```python
from build123d import *

# Parameters (mm, degrees)
SKETCH1_R               = 11.5
SKETCH1_R_2             = 10
BOSS_EXTRUDE1_DEPTH     = 6
SKETCH2_R               = 6
BOSS_EXTRUDE3_DEPTH     = 18
SKETCH4_R               = 10
CUT_EXTRUDE2_DEPTH      = 7.000000123
CUT_EXTRUDE2_DEPTH_BACK = 7.000000101
SKETCH5_R               = 4
CUT_EXTRUDE3_DEPTH      = 10
SKETCH6_R               = 4.5
SKETCH6_R_2             = 3
BOSS_EXTRUDE4_DEPTH     = 5
SKETCH7_R               = 4
CUT_EXTRUDE4_DEPTH      = 10
BOSS_EXTRUDE5_DEPTH     = 21
SKETCH9_R               = 10
CUT_EXTRUDE5_DEPTH      = 1.0000001
CUT_EXTRUDE5_DEPTH_BACK = 15.0000001
SKETCH10_R              = 1.5
CUT_EXTRUDE6_DEPTH      = 8


with BuildPart() as part:
    # Sketch1 → Boss-Extrude1 (new body, symmetric)
    with BuildSketch(Plane.XY):
        Circle(SKETCH1_R)
        Circle(SKETCH1_R_2, mode=Mode.SUBTRACT)
    extrude(amount=BOSS_EXTRUDE1_DEPTH, both=True)

    # Sketch2 → Boss-Extrude3 (add)
    with BuildSketch(Plane(origin=(0, 25, 0), x_dir=(1, 0, 0), z_dir=(0, 1, 0))):
        Circle(SKETCH2_R)
    extrude(amount=-BOSS_EXTRUDE3_DEPTH)

    # Sketch4 → Cut-Extrude2 (cut, two sides)
    with BuildSketch(Plane.XY) as cut_extrude2_sk:
        Circle(SKETCH4_R)
    extrude(amount=CUT_EXTRUDE2_DEPTH, mode=Mode.SUBTRACT)
    extrude(cut_extrude2_sk.sketch, amount=-CUT_EXTRUDE2_DEPTH_BACK, mode=Mode.SUBTRACT)

    # Sketch5 → Cut-Extrude3 (cut)
    with BuildSketch(Plane(origin=(0, 25, 0), x_dir=(1, 0, 0), z_dir=(0, 1, 0))):
        Circle(SKETCH5_R)
    extrude(amount=-CUT_EXTRUDE3_DEPTH, mode=Mode.SUBTRACT)

    # Sketch6 → Boss-Extrude4 (add)
    with BuildSketch(Plane.XY.offset(8)):
        with Locations((0, 19)):
            Circle(SKETCH6_R)
        with Locations((0, 19)):
            Circle(SKETCH6_R_2, mode=Mode.SUBTRACT)
    extrude(amount=-BOSS_EXTRUDE4_DEPTH)

    # Sketch7 → Cut-Extrude4 (cut)
    with BuildSketch(Plane(origin=(0, 25, 0), x_dir=(1, 0, 0), z_dir=(0, 1, 0))):
        Circle(SKETCH7_R)
    extrude(amount=-CUT_EXTRUDE4_DEPTH, mode=Mode.SUBTRACT)

    # Sketch8 → Boss-Extrude5 (add)
    with BuildSketch(Plane(origin=(0, 25, 0), x_dir=(1, 0, 0), z_dir=(0, 1, 0))):
        with BuildLine():
            Line((-1.5, -3.708099244), (1.5, -3.708099244))
            ThreePointArc((1.5, -3.708099244), (0, -4), (-1.5, -3.708099244))
        make_face()
    extrude(amount=-BOSS_EXTRUDE5_DEPTH)

    # Sketch9 → Cut-Extrude5 (cut, two sides)
    with BuildSketch(Plane.XY.offset(8)) as cut_extrude5_sk:
        Circle(SKETCH9_R)
    extrude(amount=CUT_EXTRUDE5_DEPTH, mode=Mode.SUBTRACT)
    extrude(cut_extrude5_sk.sketch, amount=-CUT_EXTRUDE5_DEPTH_BACK, mode=Mode.SUBTRACT)

    # Sketch10 → Cut-Extrude6 (cut)
    with BuildSketch(Plane.XY.offset(8)):
        with Locations((0, 19)):
            Circle(SKETCH10_R)
    extrude(amount=-CUT_EXTRUDE6_DEPTH, mode=Mode.SUBTRACT)


solid = part.part
```
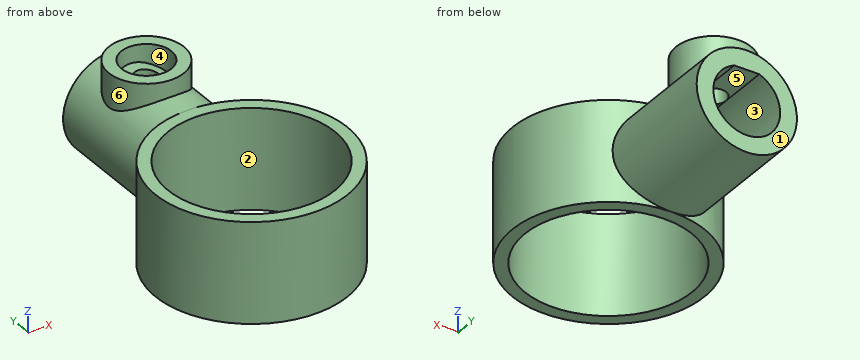
Design review of the part built by this model. Coordinates are the model's own, in mm. Face numbers are marked on the shaded views. A direction names the side the tool comes from. Give positions to 0.01 mm unless a question says otherwise; leave off trailing zeros. Order: outer loops, then holes, each group sorted by start corner. A loop starts at its lowest first (then second) coordinate and runs counter-clockwise, first axis right, second up. Notation, with made-up numbers: (55.5, -23.5) -> (62.5, -23.5) arc R32 cw to (62.5, 4.5) -> close; hole circle Ø6 at (77.5, 8). An arc over 180 degrees is marked (long way). Write each question's results on one line, items separated by ' | '. Start each with the question number.
Q1. Mouldability with a two-part tool opening along Y and no side actions: class the marked faces 1, 2, 3 and 4 as +Y half, -Y half, draft (parallel to the pull), parting line (faces both ways), or undercut.
Q2. Add section A-A on y = 0. Give the boundary of the cut face in (x, z).
Q3. Add section C-C on x = 7.25. Give the boundary of the cut face in (y, z), and give its area (3 significant figures).
Q4. Wall thickness on L1, parallel to X at y = 19, z = 4.65; L2, parallel to X at y = 0, z = 2.25; L3, parallel to Z at x = 0, y = 20.25: over which ranges is each line inside the solid? List them lowest first. Write a range as from..to.
Q5. For pin 1 (3.5 mm diameter, centred on x = 0.5, y = 16.5, fed in from -Z); pin 2 (6 mm diameter, centred on y = 15.5, z = 1, fed in from +X); pin 3 (12 mm diameter, centred on x = -8, y = 7, fed in from +Z); pin 4 (4 mm diameter, centred on x = 0, z = -1, fed in from +Y), all flat-tipped, find the tip position at first contact; note any pin that passes through.
Q6. Add section B-B on z = 0. Give the boundary of the cut face in (x, y), and give its area (3 significant figures).
Q7. Machinability: for the marked faces 5 and 6, which of the approach directions +Z, -Z, +X, -X, +Y, -Y give a long, thin tool a straight path to every point of the face, cutting with its end or side? Answer none if there is none.
Found:
1) face 1: +Y half | face 2: undercut | face 3: draft | face 4: undercut
2) outline: (-11.5, -6) -> (-10, -6) -> (-10, 6) -> (-11.5, 6) -> close; (10, -6) -> (11.5, -6) -> (11.5, 6) -> (10, 6) -> close
3) outline: (-8.93, -6) -> (-6.89, -6) -> (-6.89, 6) -> (-8.93, 6) -> close; (6.89, -6) -> (8.93, -6) -> (8.93, 6) -> (6.89, 6) -> close | area: 48.9 mm2
4) L1: x = -4.5..-1.5, 1.5..4.5 | L2: x = -11.5..-10, 10..11.5 | L3: z = -6..-4
5) pin 1: stops at z = -6 | pin 2: stops at x = 6 | pin 3: stops at z = 6 | pin 4: stops at y = 15
6) outline: (-6, 9.81) arc R11.5 ccw (long way) to (6, 9.81) -> (6, 25) -> (4, 25) -> (4, 15) -> (-4, 15) -> (-4, 25) -> (-6, 25) -> close; hole circle Ø20 at (0, 0) | area: 190 mm2
7) face 5: +Y | face 6: +Z
